Design review of the part built by this model. Coordinates are the model's own, in mm. Round coordinates to 2 decimals unless told otherwise and drop trailing zeros. Loops run counter-clockwise (first coordinate to the right, second up) from the corner with the lowest first, then second, coordinate; pieces in that order, holes last. Notation, with made-up numbers: M 1.25,-16.75 L 25.25,-16.75 A20 ccw 25.25,14.25 Z; hole C 21.5,42 d4. An arc over 180 degrees is marked long. Use a Markdown table: item, result.
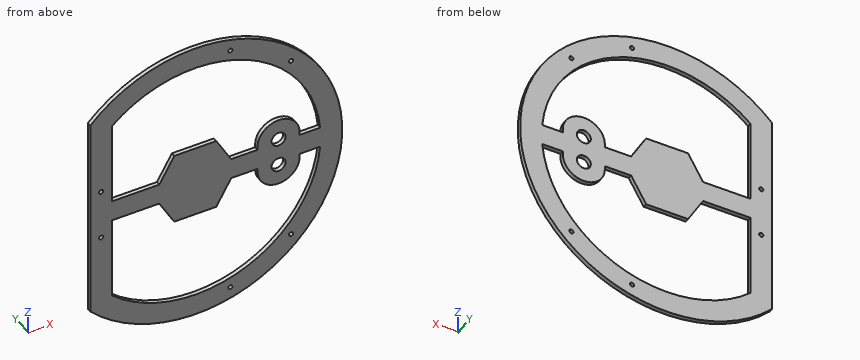
Autodesk Inventor part; units mm, degrees
ref_plane "YZ Plane" through (0, 0, 0) normal (1, 0, 0) x (0, 1, 0)
ref_plane "XZ Plane" through (0, 0, 0) normal (0, 1, 0) x (-1, 0, 0)
ref_plane "XY Plane" through (0, 0, 0) normal (0, 0, 1) x (1, 0, 0)
sketch "Sketch1" plane through (0, 0, 0) normal (0, 1, 0) x (-1, 0, 0)
  circle A0 centre (0, 0) radius 105
  line L0 (105, 0) -> (75, 0)
  line L1 (75, 0) -> (75, -73.4847)
  line L2 (75, 0) -> (75, 73.4847)
  dimension "d0" = 210
  dimension "d1" = 30
extrude "Extrusion1" add sketch "Sketch1" along normal blind 3 contours L2 L1 A0
sketch "Sketch2" plane through (0, 3, 0) normal (0, 1, 0) x (1, 0, 0)
  line L0 (-75, 73.4847) -> (-75, -73.4847)
  line L1 (-75, 0) -> (-67.25, 0)
  line L2 (-67.25, 0) -> (-67.25, -52.6096)
  line L3 (-67.25, -52.6096) -> (-67.25, 59.9001)
  line L4 (0, 0) -> (-67.25, -18.0196)
  line L5 (0, 0) -> (69.6223, 0) construction
  line L6 (0, 0) -> (-67.25, 18.0196)
  line L7 (0, 0) -> (69.6223, 0) construction
  line L8 (0, 0) -> (25.0407, -93.4533)
  line L9 (0, 0) -> (96.75, 0) construction
  line L10 (0, 0) -> (68.4126, -68.4126)
  line L11 (0, 0) -> (96.75, 0) construction
  line L12 (0, 0) -> (25.0407, 93.4533)
  line L13 (0, 0) -> (96.75, 0) construction
  line L14 (0, 0) -> (68.4126, 68.4126)
  line L15 (0, 0) -> (96.75, 0) construction
  circle A0 centre (-67.25, 18.0196) radius 1.5
  circle A1 centre (-67.25, -18.0196) radius 1.5
  circle A2 centre (25.0407, 93.4533) radius 1.5
  circle A3 centre (68.4126, 68.4126) radius 1.5
  circle A4 centre (68.4126, -68.4126) radius 1.5
  circle A5 centre (25.0407, -93.4533) radius 1.5
  dimension "d4" = 7.75
  dimension "d5" = 165
  dimension "d6" = 165
  dimension "d7" = 96.75
  dimension "d8" = 75
  dimension "d9" = 96.75
  dimension "d10" = 45
  dimension "d11" = 96.75
  dimension "d12" = 75
  dimension "d13" = 96.75
  dimension "d14" = 45
  dimension "d15" = 3
  dimension "d16" = 3
  dimension "d17" = 3
  dimension "d18" = 3
  dimension "d19" = 3
  dimension "d20" = 3
extrude "Extrusion2" cut sketch "Sketch2" against normal blind 3 contours A1 L4 L2 | L2 A1 | A0 L3 | L3 L6 A0 | L4 A1 L2 | L3 A0 L6 | A2 | A3 | A4 | A5
sketch "Sketch3" plane through (0, 3, 0) normal (0, 1, 0) x (1, 0, 0)
  circle A0 centre (-67.25, -18.0196) radius 1.5
  line L0 (-67.25, -18.0196) -> (-75, -18.0196)
  line L1 (-75, 73.4847) -> (-75, -73.4847)
  line L2 (-75, -18.0196) -> (-59.5, -18.0196)
  line L3 (-59.5, -18.0196) -> (-59.5, -66.8581)
  line L4 (-59.5, -18.0196) -> (-59.5, 66.8581)
  arc A1 (-59.5, -66.8581) -> (-59.5, 66.8581) centre (0, 0) ccw
  point P0 (0, 0)
  dimension "d23" = 15.5
extrude "Extrusion3" cut sketch "Sketch3" against normal blind 3 contours L4 A1 L3
sketch "Sketch4" plane through (0, 3, 0) normal (0, 1, 0) x (1, 0, 0)
  arc A0 (-59.5, -66.8581) -> (-59.5, 66.8581) centre (0, 0) ccw
  line L0 (89.5, 0) -> (59.5, 0)
  line L1 (59.5, 0) -> (59.5, 10)
  line L2 (59.5, 10) -> (59.5, -10)
  circle A1 centre (59.5, -10) radius 5
  circle A2 centre (59.5, 10) radius 5
  circle A3 centre (59.5, 10) radius 15
  circle A4 centre (59.5, -10) radius 15
  line L3 (44.5, -10) -> (44.5, 10)
  line L4 (74.5, 10) -> (74.5, -10)
  point P0 (0, 0)
  dimension "d27" = 30
  dimension "d28" = 10
  dimension "d29" = 20
  dimension "d30" = 10
  dimension "d31" = 10
extrude "Extrusion4" add sketch "Sketch4" against normal blind 3
sketch "Sketch5" plane through (0, 3, 0) normal (0, 1, 0) x (1, 0, 0)
  line L0 (44.5, -10) -> (44.5, 10)
  line L1 (44.5, 0) -> (-59.5, 0)
  line L2 (-59.5, 66.8581) -> (-59.5, -66.8581)
  line L3 (-41.4459, 0) -> (-41.4459, 7.5)
  line L4 (-41.4459, 7.5) -> (-41.4459, -7.5)
  line L5 (-41.4459, -7.5) -> (-59.5, -7.5)
  line L6 (-41.4459, -7.5) -> (44.5, -7.5)
  line L7 (-41.4459, 7.5) -> (-59.5, 7.5)
  line L8 (-41.4459, 7.5) -> (44.5, 7.5)
  point P0 (0, 0)
  dimension "d34" = 7.5
  dimension "d35" = 15
extrude "Extrusion5" add sketch "Sketch5" against normal blind 3 contours L1 L3 L8 L0 | L5 L2 L1 L4 | L1 L2 L7 L3
sketch "Sketch6" plane through (0, 3, 0) normal (0, 1, 0) x (1, 0, 0)
  line L0 (-41.4459, -7.5) -> (-41.4459, 0)
  line L1 (-41.4459, 0) -> (44.5, 0)
  line L2 (-41.4459, -7.5) -> (44.5, -7.5)
  line L3 (44.5, -7.5) -> (44.5, 0)
  line L4 (44.5, 0) -> (-41.4459, 0)
  line L5 (-41.4459, 0) -> (-41.4459, -7.5)
  point P0 (0, 0)
extrude "Extrusion6" add sketch "Sketch6" against normal blind 3
sketch "Sketch7" plane through (0, 3, 0) normal (0, 1, 0) x (1, 0, 0)
  line L0 (44.5, -7.5) -> (-59.5, -7.5)
  line L1 (74.5, 10) -> (74.5, -10)
  line L2 (44.5, -7.5) -> (74.5, -7.5)
  line L3 (74.5, -7.5) -> (74.5, 7.5)
  line L4 (74.5, 7.5) -> (44.5, 7.5)
  line L5 (44.5, 7.5) -> (44.5, -7.5)
  line L6 (74.5, 7.5) -> (92.1337, 7.5)
  line L7 (92.1337, 7.5) -> (92.1337, -7.5)
  line L8 (92.1337, -7.5) -> (74.5, -7.5)
  line L9 (74.5, -7.5) -> (74.5, 7.5)
  point P0 (0, 0)
  dimension "d40" = 15
extrude "Extrusion7" add sketch "Sketch7" against normal blind 3 contours L6 L7 L8 L1
sketch "Sketch8" plane through (0, 3, 0) normal (0, 1, 0) x (1, 0, 0)
  line L0 (0, 0) -> (-30, 0)
  line L1 (0, 0) -> (-15, 25.9808)
  line L2 (0, 0) -> (30, 0) construction
  line L3 (-15, 25.9808) -> (-30, 0)
  line L4 (0, 0) -> (15, 25.9808)
  line L5 (15, 25.9808) -> (-15, 25.9808)
  line L6 (0, 0) -> (30, 0)
  line L7 (30, 0) -> (15, 25.9808)
  line L8 (0, 0) -> (15, -25.9808)
  line L9 (15, -25.9808) -> (30, 0)
  line L10 (0, 0) -> (-15, -25.9808)
  line L11 (-15, -25.9808) -> (15, -25.9808)
  line L12 (-15, -25.9808) -> (-30, 0)
  dimension "d43" = 30
  dimension "d44" = 30
  dimension "d45" = 120
extrude "Extrusion8" add sketch "Sketch8" against normal blind 3 contours L10 L12 L0 | L0 L3 L1 | L4 L7 L6 | L6 L9 L8 | L8 L11 L10
sketch "Sketch9" plane through (0, 3, 0) normal (0, 1, 0) x (1, 0, 0)
  line L0 (4.3301, 7.5) -> (15, 25.9808)
  line L1 (-25.6699, 7.5) -> (-15, 25.9808)
  line L2 (15, 25.9808) -> (-15, 25.9808)
  line L3 (-15, 25.9808) -> (-4.3301, 7.5)
  line L4 (-15, 25.9808) -> (-4.3301, 7.5)
  line L5 (-4.3301, 7.5) -> (4.3988, 7.5)
  line L6 (-4.3301, 7.5) -> (4.3301, 7.5)
  line L7 (25.6699, 7.5) -> (15, 25.9808)
  line L8 (4.3301, 7.5) -> (15, 25.9808)
  point P0 (0, 0)
extrude "Extrusion9" add sketch "Sketch9" against normal blind 3
properties part number "Top Plate1"
1. Take a section at D-D on y = 0.8. Count the separate pieces of the cut face and the enclosed holes in it, and give its area (3 significant figures).
Check values:
| item | result |
|---|---|
| separate pieces | 1 |
| enclosed holes | 10 |
| area | 13,600 mm² |
2. Take a section at B-B on z = -76. Give the boundary of the cut face in (x, y), and give its area (3 significant figures).
Check values:
| item | result |
|---|---|
| outline | M -72.45,0 L -47.27,0 L -47.27,3 L -72.45,3 Z; M 47.27,0 L 72.45,0 L 72.45,3 L 47.27,3 Z |
| area | 151 mm² |
3. Take a section at A-A on x = 59.5. Give the boundary of the cut face in (y, z), and give its area (3 significant figures).
Check values:
| item | result |
|---|---|
| outline | M 0,-86.51 L 3,-86.51 L 3,-66.86 L 0,-66.86 Z; M 0,-25 L 3,-25 L 3,-15 L 0,-15 Z; M 0,-5 L 3,-5 L 3,5 L 0,5 Z; M 0,15 L 3,15 L 3,25 L 0,25 Z; M 0,66.86 L 3,66.86 L 3,86.51 L 0,86.51 Z |
| area | 208 mm² |
4. Take a section at C-C on x = 32. Give the boundary of the cut face in (y, z) (3 decimals).
Check values:
| item | result |
|---|---|
| outline | M 0,-100.005 L 3,-100.005 L 3,-83.584 L 0,-83.584 Z; M 0,-7.5 L 3,-7.5 L 3,7.5 L 0,7.5 Z; M 0,83.584 L 3,83.584 L 3,100.005 L 0,100.005 Z |
5. Wall thickness on line 1 along Z through (x, y) = (37.5, 1.95); line 2 along Z through (x, y) = (43, 1.4); line 3 along Z through (x, y) = (59.5, 1.05): over which ranges is each line inside the solid? List them lowest first. Write a range as from..to.
Check values:
| item | result |
|---|---|
| line 1 | z = -98.08..-81.27, -7.5..7.5, 81.27..98.08 |
| line 2 | z = -95.79..-78.49, -7.5..7.5, 78.49..95.79 |
| line 3 | z = -86.51..-66.86, -25..-15, -5..5, 15..25, 66.86..86.51 |
6. Insertion check: pin 1 (6 mm diameter, centred on x = 59.5, z = -10, fed in from +Y); pin 2 (0.9 mm diameter, centred on x = -36, y = 1.5, fed in from +Z); pin 3 (5 mm diameter, centred on x = 25.04, z = 93.45, fed in from -Y). Each pin has a flat end and moves straight along its axis. Give the tip position at first contact, or say it passes through.
Check values:
| item | result |
|---|---|
| pin 1 | passes through |
| pin 2 | stops at z = 98.8 |
| pin 3 | stops at y = 0 |
